Autodesk Inventor part; units mm, degrees
ref_plane "YZ Plane" through (0, 0, 0) normal (1, 0, 0) x (0, 1, 0)
ref_plane "XZ Plane" through (0, 0, 0) normal (0, 1, 0) x (-1, 0, 0)
ref_plane "XY Plane" through (0, 0, 0) normal (0, 0, 1) x (1, 0, 0)
sketch "Sketch1" plane through (0, 0, 0) normal (0, 0, 1) x (1, 0, 0)
  circle A0 centre (31.1774, 0) radius 8 construction
  circle A1 centre (0, 0) radius 8 construction
  line L0 (7.5887, 10.3156) -> (11.7298, -5.1392) construction
  line L1 (11.7298, -5.1392) -> (2.0706, -7.7274)
  line L2 (-2.0706, 7.7274) -> (7.5887, 10.3156)
  line L3 (19.4476, -5.1392) -> (23.5887, 10.3156) construction
  line L4 (23.5887, 10.3156) -> (33.248, 7.7274)
  line L5 (19.4476, -5.1392) -> (29.1069, -7.7274)
  line L6 (7.5887, 10.3156) -> (23.5887, 10.3156) construction
  line L7 (11.7298, -5.1392) -> (19.4476, -5.1392)
  arc A2 (-2.0706, 7.7274) -> (2.0706, -7.7274) centre (0, 0) ccw
  arc A3 (29.1069, -7.7274) -> (33.248, 7.7274) centre (31.1774, 0) ccw
  arc A4 (23.5887, 10.3156) -> (7.5887, 10.3156) centre (15.5887, -19.5408) ccw
  point P0 (15.5887, 10.3156)
  dimension "d0" = 16
  dimension "d1" = 16
  dimension "d2" = 16
  dimension "d3" = 10
  dimension "d4" = 10
  dimension "d5" = 16
  dimension "d6" = 16
  dimension "d7" = 75
extrude "Extrusion1" add sketch "Sketch1" along normal blind 46
sketch "Sketch2" plane through (0, 0, 46) normal (0, 0, 1) x (1, 0, 0)
  arc A0 (-2.0706, 7.7274) -> (2.0706, -7.7274) centre (0, 0) ccw
  arc A1 (29.1069, -7.7274) -> (33.248, 7.7274) centre (31.1774, 0) ccw
  line L0 (11.7298, -5.1392) -> (19.4476, -5.1392)
  circle A2 centre (0, 0) radius 1.75
  circle A3 centre (31.1774, 0) radius 1.75
  circle A4 centre (15.5887, 7.8608) radius 1.75
  point P0 (0, 0)
  point P1 (15.5887, -5.1392)
  dimension "d11" = 3.5
  dimension "d12" = 3.5
  dimension "d13" = 3.5
  dimension "d14" = 13
extrude "Extrusion2" cut sketch "Sketch2" against normal through all
sketch "Sketch3" plane through (0, 0, 46) normal (0, 0, 1) x (1, 0, 0)
  arc A0 (23.5887, 10.3156) -> (7.5887, 10.3156) centre (15.5887, -19.5408) ccw
  line L0 (7.5887, 10.3156) -> (23.5887, 10.3156)
  line L1 (19.4476, -5.1392) -> (29.1069, -7.7274)
  line L2 (23.5887, 10.3156) -> (19.4476, -5.1392)
  line L3 (11.7298, -5.1392) -> (19.4476, -5.1392)
  line L4 (19.4476, -5.1392) -> (11.7298, -5.1392)
  line L5 (11.7298, -5.1392) -> (7.5887, 10.3156)
  circle A1 centre (15.5887, 7.8608) radius 1.75
  point P0 (0, 0)
extrude "Extrusion3" add sketch "Sketch3" along normal blind 16
sketch "Sketch4" plane through (0, 0, 62) normal (0, 0, 1) x (1, 0, 0)
  arc A0 (23.5887, 10.3156) -> (7.5887, 10.3156) centre (15.5887, -19.5408) ccw construction
  line L0 (7.5887, 10.3156) -> (23.5887, 10.3156) construction
  line L1 (23.5887, 10.3156) -> (15.5887, 10.3156) construction
  line L2 (11.7298, -5.1392) -> (19.4476, -5.1392) construction
  line L3 (15.5887, -5.1392) -> (15.5887, 10.3156) construction
  circle A1 centre (15.5887, 2.5882) radius 1.5
  point P0 (0, 0)
  dimension "d19" = 3
extrude "Extrusion4" cut sketch "Sketch4" against normal through all
sketch "Sketch7" plane through (0, 0, 0) normal (0, 1, 0) x (-1, 0, 0)
  circle A0 centre (-26.5887, 38) radius 1.5
  circle A1 centre (-4.5887, 38) radius 1.5
  line L0 (-7.5887, 62) -> (-23.5887, 62) construction
  line L1 (-26.5887, 38) -> (-4.5887, 38) construction
  point P0 (0, 0)
  point P1 (-15.5887, 62)
  point P2 (-15.5887, 38)
  dimension "d28" = 3
  dimension "d29" = 3
  dimension "d30" = 22
  dimension "d31" = 24
extrude "Extrusion7" cut sketch "Sketch7" along normal through all
properties material "ABS Plastic"
Geometry: final body of the model. Coordinates: model frame, mm. A direction names the side the tool comes from. Round coordinates to 2 decimals unless told otherwise and drop trailing zeros. Write each loop counter-clockwise with the first axis right and the second up, starting at its lowest first coordinate (ties: lowest second). Pieces come first, ordered by that corner, then holes. Notation, with made-up numbers: (78.25, 4.25) -> (108.25, 4.25) arc R7 cw to (108.25, 12.25) -> close; hole circle Ø3 at (81, 82.25). An arc over 180 degrees is marked (long way). Use CSV: the item, a comma, the result in double quotes. Start each with the question number.
Q1. Section D-D (x = 15.5). Return loops of the section in (y, z), plus the area to 3 significant figures.
Q2. Pull-direction query (X, two-part tool) for faces 6 (the face through (9.69, 2.48, 53.89)), 7 (the face through (2, 1, 46)), 8 (the face through (28.35, 9.04, 22.68)), 9 (the face through (27, 0, 38)); classes: pulls with the +X half, pulls with the -X half, needs draft (parallel to the pull), parting line crosses it, or undercut.
Q3. First-contact query: pin 1 Ø1.5 at (x, z) = (5, 54.5) entering from -Y; pin 2 Ø3 at (x, z) = (2.5, 32) entering from +Y; pin 3 Ø6 at (x, z) = (2.5, 36) entering from +Y; pin 4 Ø3 at (y, z) = (4.5, 32.5) entering from -X. Flat tips, straight axial feed; report the tip coordinate or a pass-through.
Q4. Section A-A (x = 0). Return loops of the section in (y, z), plus the area to 3 significant figures.
Q5. Reachability of faces 1 (the face through (6.968, -6.415, 22.678)), 2 (the face through (5, 0, 38)), 3 (the face through (15, 5, 62)), 4 (the face through (29, 1, 46)), 5 (the face through (14.09, 2.65, 31.43)) from +Z, -Z, +X, -X, +Y, -Y: full face, straight path, thin tool, end or side. Return the list, or none.
Q6. Section B-B (y = 5). Return loops of the section in (x, z) (3 decimals).
Q7. Section C-C (z = 38). Return loops of the section in (x, y), plus the area to 3 significant figures.
Q8. Line query: L1, parallel to Y at x = 15.5, z = 42; L2, parallel to Y at x = 16, z = 36.5; L3, parallel to X at y = 6.5, z = 38. Output: solid intervals per line, ascending.
Result sheet:
1,outline,"(-5.14, 0) -> (1.09, 0) -> (1.09, 62) -> (-5.14, 62) -> close; (4.09, 0) -> (6.11, 0) -> (6.11, 62) -> (4.09, 62) -> close; (9.61, 0) -> (11.37, 0) -> (11.37, 62) -> (9.61, 62) -> close"
1,area,"621 mm²"
2,face 6,"pulls with the -X half"
2,face 7,"needs draft"
2,face 8,"pulls with the +X half"
2,face 9,"undercut"
3,pin 1,"through"
3,pin 2,"y = 9.35"
3,pin 3,"y = 9.76"
3,pin 4,"x = -7.42"
4,outline,"(-8, 0) -> (-1.75, 0) -> (-1.75, 46) -> (-8, 46) -> close; (1.75, 0) -> (8.28, 0) -> (8.28, 46) -> (1.75, 46) -> close"
4,area,"588 mm²"
5,face 1,"+Z, -Z, -Y"
5,face 2,"+Y"
5,face 3,"+Z, +X, -X, +Y, -Y"
5,face 4,"+Z, +X, -Y"
5,face 5,"+Z, -Z"
6,outline,"(-6.245, 0) -> (37.422, 0) -> (37.422, 46) -> (22.164, 46) -> (22.164, 62) -> (9.013, 62) -> (9.013, 46) -> (-6.245, 46) -> close; hole circle Ø3 at (4.589, 38); hole circle Ø3 at (26.589, 38)"
7,outline,"(-2.07, 7.73) arc R8 ccw to (2.07, -7.73) -> (11.73, -5.14) -> (19.45, -5.14) -> (29.11, -7.73) arc R8 ccw to (33.25, 7.73) -> (28.09, 9.11) -> (28.09, 0) -> (25.09, 0) -> (25.09, 9.91) -> (23.59, 10.32) arc R30.91 ccw to (7.59, 10.32) -> (6.09, 9.91) -> (6.09, 0) -> (3.09, 0) -> (3.09, 9.11) -> close; hole circle Ø3.5 at (0, 0); hole circle Ø3.5 at (15.59, 7.86); hole circle Ø3 at (15.59, 2.59); hole circle Ø3.5 at (31.18, 0)"
7,area,"623 mm²"
8,L1,"-5.14 to 1.09, 4.09 to 6.11, 9.61 to 11.37"
8,L2,"-5.14 to 1.15, 4.03 to 6.16, 9.56 to 11.37"
8,L3,"-4.66 to 3.09, 6.09 to 14.49, 16.69 to 25.09, 28.09 to 35.84"
